Answer from the drawing. Dimensions are ordinates in mm from the lowest x, y and z of the part. Coordinates: 2 decimals unless noted, no trailing zeros. Order: outer loops, then holes, each group sorted by start corner. A loop starts at its lowest first (then second) coordinate and runs counter-clockwise, first axis right, second up. Notation, with made-up numbers: (-30.75, 25.25) -> (25.25, 25.25) arc R19 ccw to (25.25, 41.25) -> close; hole circle Ø10 at (48.25, 56). An arc over 180 degrees is marked (long way). Answer in a Markdown table with one row per item.
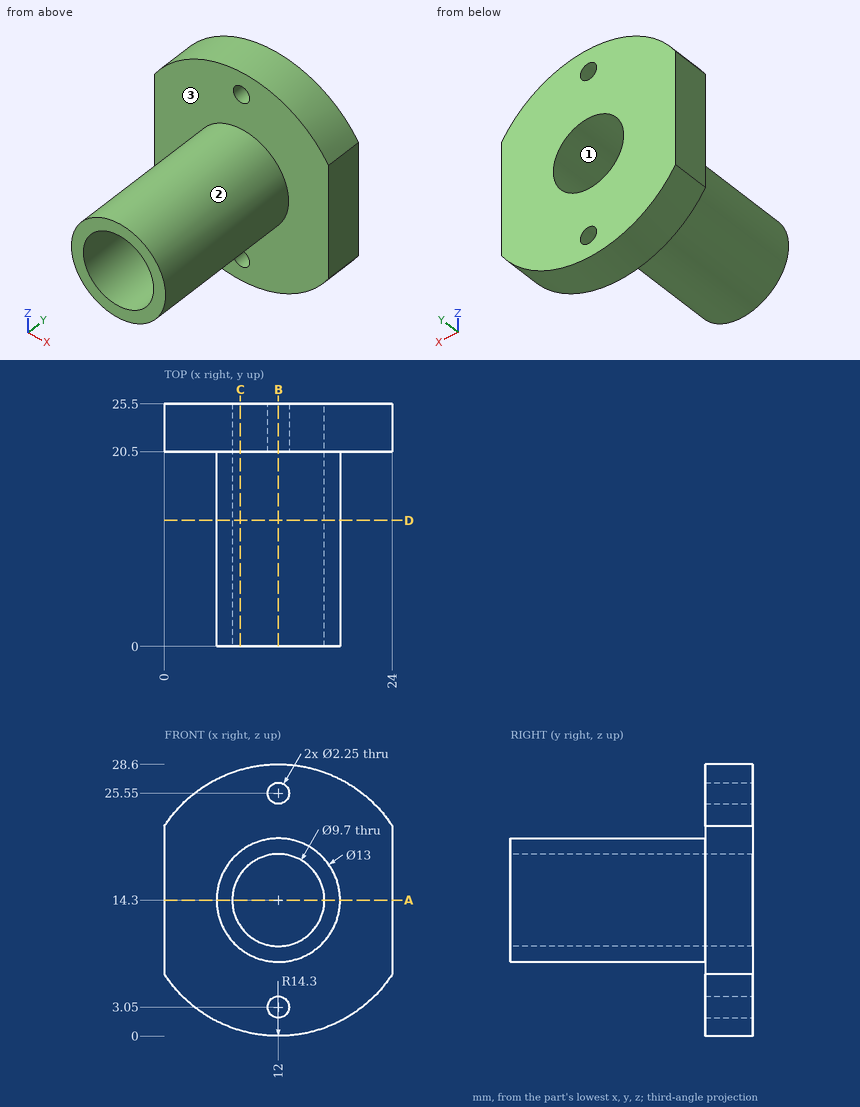
Q1. Consider line 1 (Z direction, x = 12, y = 24) (3 decimals); line 2 (Z direction, x = 12, y = 11.5); line 3 (Y direction, x = 12.25, z = 24.25). Determine where each line is inside the solid, lowest interval first.
Outcome:
| item | result |
|---|---|
| line 1 | 0 to 1.925, 4.175 to 9.45, 19.15 to 24.425, 26.675 to 28.6 |
| line 2 | 7.8 to 9.45, 19.15 to 20.8 |
| line 3 | 20.5 to 25.5 |
Q2. The part is cut by section C-C (x = 8). Write down the section's boundary in (y, z), then the cut area to 3 significant figures.
Outcome:
| item | result |
|---|---|
| outline | (0, 9.18) -> (20.5, 9.18) -> (20.5, 0.57) -> (25.5, 0.57) -> (25.5, 11.56) -> (0, 11.56) -> close; (0, 17.04) -> (25.5, 17.04) -> (25.5, 28.03) -> (20.5, 28.03) -> (20.5, 19.42) -> (0, 19.42) -> close |
| area | 207 mm² |
Q3. Given pin 1 (1.3 mm diameter, centred on x = 12, z = 25.55, fed in from +Y); pin 2 (1 mm diameter, centred on x = 16, z = 5.5, fed in from -Y); pin 3 (1.5 mm diameter, centred on y = 19, z = 13.5, fed in from +X); pin 4 (5 mm diameter, centred on x = 10.5, y = 9.5, fed in from -Z), each flat-ended and moving along its own axis, determine where each tip first touches the part or whether it passes through.
Outcome:
| item | result |
|---|---|
| pin 1 | through |
| pin 2 | y = 20.5 |
| pin 3 | x = 18.5 |
| pin 4 | z = 7.8 |
Q4. The part is cut by section B-B (x = 12). Write down the section's boundary in (y, z) (3 decimals).
Outcome:
| item | result |
|---|---|
| outline | (0, 7.8) -> (20.5, 7.8) -> (20.5, 4.175) -> (25.5, 4.175) -> (25.5, 9.45) -> (0, 9.45) -> close; (0, 19.15) -> (25.5, 19.15) -> (25.5, 24.425) -> (20.5, 24.425) -> (20.5, 20.8) -> (0, 20.8) -> close; (20.5, 0) -> (25.5, 0) -> (25.5, 1.925) -> (20.5, 1.925) -> close; (20.5, 26.675) -> (25.5, 26.675) -> (25.5, 28.6) -> (20.5, 28.6) -> close |
Q5. For a pull along Z with two mould halves and no side action, classify the marked faces 1, 2 and 3 as pulls with the +Z half, pulls with the -Z half, needs draft (parallel to the pull), parting line crosses it, or undercut.
Outcome:
| item | result |
|---|---|
| face 1 | undercut |
| face 2 | parting line crosses it |
| face 3 | needs draft |
Q6. The part is cut by section D-D (y = 13.25). Write down the section's boundary in (x, z).
Outcome:
| item | result |
|---|---|
| outline | circle Ø13 at (12, 14.3); hole circle Ø9.7 at (12, 14.3) |
Q7. The part is cut by section A-A (z = 14.3). Write down the section's boundary in (x, y), then the cut area to 3 significant figures.
Outcome:
| item | result |
|---|---|
| outline | (0, 20.5) -> (5.5, 20.5) -> (5.5, 0) -> (7.15, 0) -> (7.15, 25.5) -> (0, 25.5) -> close; (16.85, 0) -> (18.5, 0) -> (18.5, 20.5) -> (24, 20.5) -> (24, 25.5) -> (16.85, 25.5) -> close |
| area | 139 mm² |
